from build123d import *

# Parameters (mm, degrees)
SKETCH_1_W               = 90
SKETCH_1_H               = 3
EXTRUDE_1_DEPTH          = 3
EXTRUDE_1_DEPTH_BACK     = 3
SKETCH_2_W               = 40
SKETCH_2_H               = 6
CUT_EXTRUDE_1_DEPTH      = 5
CUT_EXTRUDE_5_DEPTH      = 1
CUT_EXTRUDE_5_DEPTH_BACK = 3
SKETCH_4_OUTSIDE_W       = 111.734
SKETCH_4_OUTSIDE_H       = 27.734
SKETCH_4_OUTSIDE_R       = 3


with BuildPart() as part:
    # 草图1 → 旋转1 (revolve)
    with BuildSketch(Plane.XY, mode=Mode.PRIVATE) as revolve_1_sk:
        with Locations((-1.966019417, 1.5)):
            Rectangle(SKETCH_1_W, SKETCH_1_H)
    revolve(revolve_1_sk.sketch.rotate(Axis((-46.966019417, 0, 0), (1, 0, 0)), 90), axis=Axis((-46.966019417, 0, 0), (1, 0, 0)))

    # 草图2 → 凸台-拉伸1 (add, two sides: drawn at the far end of the back side and taken through both)
    with BuildSketch(Plane(origin=(0, 0, 0), x_dir=(0, 0, -1), z_dir=(1, 0, 0)).offset(-EXTRUDE_1_DEPTH_BACK)):
        Rectangle(SKETCH_2_W, SKETCH_2_H)
    extrude(amount=EXTRUDE_1_DEPTH + EXTRUDE_1_DEPTH_BACK)

    # 草图3 → 切除-拉伸1 (cut)
    with BuildSketch(Plane(origin=(0, 0, -20), x_dir=(-1, 0, 0), z_dir=(0, 0, -1))):
        with BuildLine():
            Line((-3, 3), (-3, 0))
            ThreePointArc((-3, 0), (-2.121320344, 2.121320344), (0, 3))
            Line((0, 3), (-3, 3))
        make_face()
        with BuildLine():
            ThreePointArc((0, 3), (2.121320344, 2.121320344), (3, 0))
            Line((3, 0), (3, 3))
            Line((3, 3), (0, 3))
        make_face()
        with BuildLine():
            Line((-3, -3), (0, -3))
            ThreePointArc((0, -3), (-2.121320344, -2.121320344), (-3, 0))
            Line((-3, 0), (-3, -3))
        make_face()
        with BuildLine():
            Line((0, -3), (3, -3))
            Line((3, -3), (3, 0))
            ThreePointArc((3, 0), (2.121320344, -2.121320344), (0, -3))
        make_face()
    extrude(amount=-CUT_EXTRUDE_1_DEPTH, mode=Mode.SUBTRACT)

    # 草图4 outside → 切除-拉伸5 (cut, two sides: drawn at the far end of the back side and taken through both)
    with BuildSketch(Plane.XY.offset(8).offset(-CUT_EXTRUDE_5_DEPTH_BACK)):
        with Locations((-1.966, 0)):
            Rectangle(SKETCH_4_OUTSIDE_W, SKETCH_4_OUTSIDE_H)
        with Locations(Location((0, 0, 0), (0, 0, 180))):
            Circle(SKETCH_4_OUTSIDE_R, mode=Mode.SUBTRACT)
    extrude(amount=CUT_EXTRUDE_5_DEPTH + CUT_EXTRUDE_5_DEPTH_BACK, mode=Mode.SUBTRACT)


solid = part.part
Geometry check sheet. Reference: the model listing, model coordinates, mm. A direction names the side the tool comes from. Round coordinates to 2 decimals unless told otherwise and drop trailing zeros. Order: outer loops, then holes, each group sorted by start corner. A loop starts at its lowest first (then second) coordinate and runs counter-clockwise, first axis right, second up. Notation, with made-up numbers: M -14,-9.5 L -1,-9.5 A33 cw -1,21.5 Z; hole C -8.75,-19.75 d3. An arc over 180 degrees is marked long. Answer in a Markdown table with one row per item.
(1) Sectioned sample at A-A, the plane y = -0.9. Record the cut outline in (x, z).
Responses:
| item | result |
|---|---|
| outline | M -46.97,-2.86 L -3,-2.86 L -3,-15 L -2.86,-15 L -2.86,-20 L 2.86,-20 L 2.86,-15 L 3,-15 L 3,-2.86 L 43.03,-2.86 L 43.03,2.86 L 3,2.86 L 3,5 L 2.86,5 L 2.86,9 L 3,9 L 3,20 L -3,20 L -3,9 L -2.86,9 L -2.86,5 L -3,5 L -3,2.86 L -46.97,2.86 Z |
(2) Sectioned sample at B-B, the plane z = -4. Record the cut outline in (x, y).
Responses:
| item | result |
|---|---|
| outline | M -3,-3 L 3,-3 L 3,3 L -3,3 Z |
(3) Sectioned sample at C-C, the plane x = -19. Record the cut outline in (y, z), and give its area (3 significant figures).
Responses:
| item | result |
|---|---|
| outline | C 0,0 d6 |
| area | 28.3 mm² |
(4) Go/stop test with flat-tipped pins: P1, Ø1, axis at x = -36, y = -0.5, coming from the -Z side; P2, Ø1.5, axis at x = 28.5, y = 0, coming from the +Z side; P3, Ø5, axis at x = -7.5, z = 3.5, coming from the +Y side. Record where each tip stops, or that it passes through.
Responses:
| item | result |
|---|---|
| P1 | stops at z = -3 |
| P2 | stops at z = 3 |
| P3 | stops at y = 2.83 |
(5) Scan lines: probe 1 along X at (y, z) = (2.2, -5.5); probe 2 along Z at (x, y) = (-41.5, -0.6). Record each from-to range of solid material in increasing order. Write a range as from..to.
Responses:
| item | result |
|---|---|
| probe 1 | x = -3..3 |
| probe 2 | z = -2.94..2.94 |
(6) Draft check along Z on faces 5 (the face through (-2.4, 2.3, 5)), 6 (the face through (3, 0, 15)), 7 (the face through (23.3, -0.9, 2.86)), 8 (the face through (2.4, 2.3, -15)). Enter one of: released by +Z, released by -Z, zero draft, split by the parting line, or undercut.
Responses:
| item | result |
|---|---|
| face 5 | undercut |
| face 6 | zero draft |
| face 7 | split by the parting line |
| face 8 | released by -Z |
(7) Tool access check on faces 1 (the face through (-2.4, -2.3, 9)), 2 (the face through (2.3, 2.4, 5)), 3 (the face through (-2.86, -0.9, 6.97)), 4 (the face through (-2.4, 2.3, 9)). Record the directions out of +Z, -Z, +X, -X, +Y, -Y that give a thin tool (end or side, any length) a straight path to the whole face; none if there is none.
Responses:
| item | result |
|---|---|
| face 1 | -X, -Y |
| face 2 | +X, +Y |
| face 3 | none |
| face 4 | -X, +Y |
